Check sheet for the drawn part. Datum: minimum x, y, z corner. Units: mm. Give positions to 0.01 mm unless a question says otherwise; leave off trailing zeros. Loops run counter-clockwise (first coordinate to the right, second up) from the corner with the lowest first, then second, coordinate; pieces in that order, holes last. Notation, with made-up numbers: (40.25, 38.25) - (76.25, 38.25) arc R19 ccw to (76.25, 67.25) - close; hole circle Ø10 at (31.25, 2.5). An arc over 180 degrees is marked (long way). Use a Markdown table: item, result. Add a question column.
1. Depth check by flat-ended pin: P1, Ø4, axis at x = 59, y = 5.5, coming from the +Z side; P2, Ø2, axis at x = 40.5, y = 1.5, coming from the -Z side; P3, Ø4.5, axis at x = 61.5, z = 160.5, coming from the +Y side; P4, Ø1.2, axis at y = 3, z = 160, coming from the +X side. Enter the tip coordinate at first touch or a pass-through.
2. Cross-section at C-C on x = 88. Enter the section's corners in (y, z).
3. Cross-section at B-B on z = 83. Enter the section's corners in (x, y), and give its area (3 significant figures).
4. Cross-section at A-A on y = 6. Enter the section's corners in (x, z) (1 decimal).
5. Material ranges on L1, parallel to Z at x = 49, y = 7.75; L2, parallel to X at y = 5.25, z = 33 (1 decimal); L3, parallel to X at y = 1.5, z = 130, recorded low to high.
6. Cross-section at D-D on x = 72.5. Enter the section's corners in (y, z) (1 decimal).
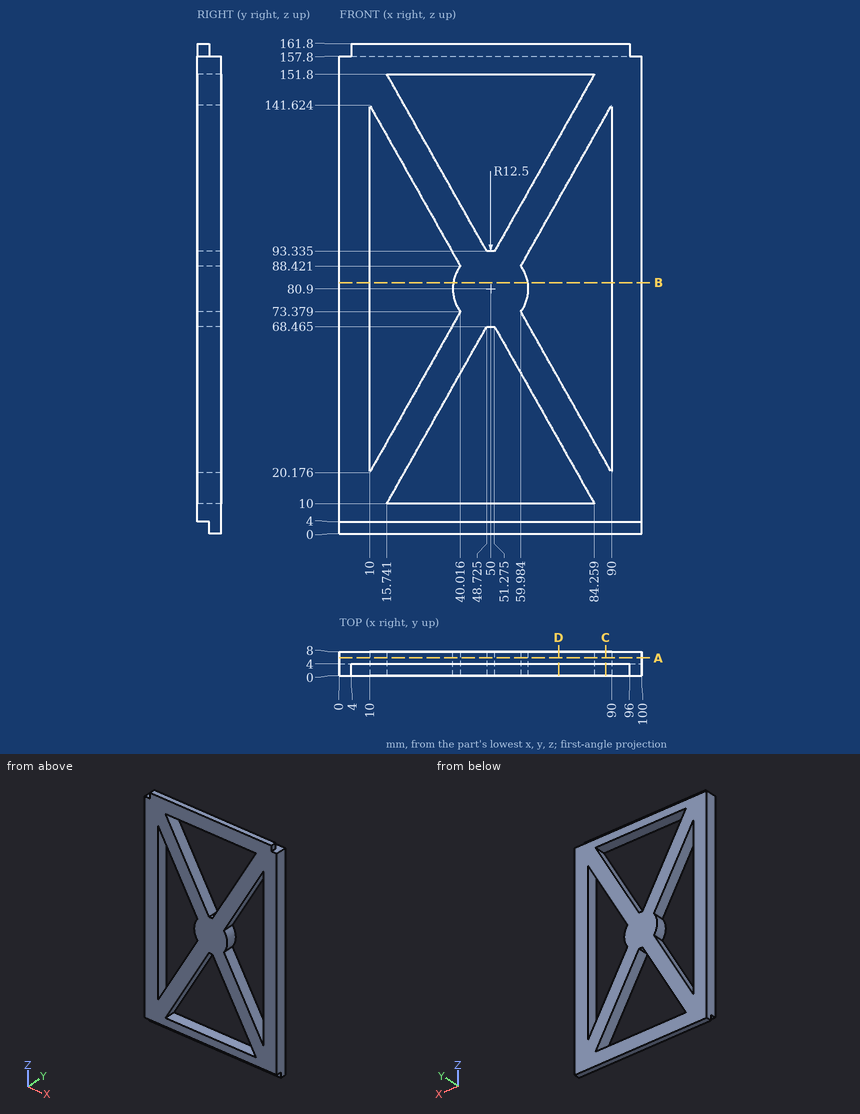
Values found:
| question | item | result |
|---|---|---|
| 1 | P1 | stops at z = 161.8 |
| 1 | P2 | stops at z = 4 |
| 1 | P3 | stops at y = 4 |
| 1 | P4 | stops at x = 96 |
| 2 | outline | (0, 4) - (4, 4) - (4, 0) - (8, 0) - (8, 23.72) - (0, 23.72) - close; (0, 138.08) - (8, 138.08) - (8, 157.8) - (4, 157.8) - (4, 161.8) - (0, 161.8) - close |
| 3 | outline | (0, 0) - (10, 0) - (10, 8) - (0, 8) - close; (37.68, 0) - (62.32, 0) - (62.32, 8) - (37.68, 8) - close; (90, 0) - (100, 0) - (100, 8) - (90, 8) - close |
| 3 | area | 357 mm2 |
| 4 | outline | (0, 0) - (100, 0) - (100, 157.8) - (0, 157.8) - close; hole (10, 20.2) - (40, 73.4) arc R12.5 cw to (40, 88.4) - (10, 141.6) - close; hole (15.7, 10) - (84.3, 10) - (51.3, 68.5) arc R12.5 cw to (48.7, 68.5) - close; hole (15.7, 151.8) - (48.7, 93.3) arc R12.5 cw to (51.3, 93.3) - (84.3, 151.8) - close; hole (60, 73.4) - (90, 20.2) - (90, 141.6) - (60, 88.4) arc R12.5 cw to start |
| 5 | L1 | z = 0 to 10, 68.44 to 93.36, 151.8 to 157.8 |
| 5 | L2 | x = 0 to 10, 17.2 to 28.7, 71.3 to 82.8, 90 to 100 |
| 5 | L3 | x = 0 to 10, 16.56 to 28.04, 71.96 to 83.44, 90 to 100 |
| 6 | outline | (0, 4) - (4, 4) - (4, 0) - (8, 0) - (8, 10) - (0, 10) - close; (0, 30.8) - (8, 30.8) - (8, 51.2) - (0, 51.2) - close; (0, 110.6) - (8, 110.6) - (8, 131) - (0, 131) - close; (0, 151.8) - (8, 151.8) - (8, 157.8) - (4, 157.8) - (4, 161.8) - (0, 161.8) - close |
